Read the model definition and answer for the solid it produces. Units are mm, in the model's axes. Face numbers are marked on the shaded views. A direction names the side the tool comes from. Coordinates: 2 decimals unless noted, no trailing zeros. Loops run counter-clockwise (first coordinate to the right, second up) from the corner with the lowest first, then second, coordinate; pieces in that order, holes last.
Q1. Which of the six approach directions +Z, -Z, +X, -X, +Y, -Y give full straight-line access (tool end or side, diameter ignored) to the marked faces 1 and 2?
Q2. Section B-B (x = 2) is taken. Give the vertices of the cut face in (y, z), then the cut area to 4 significant figures.
Q3. Section A-A (y = 18.25) is taken. Give the vertices of the cut face in (x, z).
Q4. Straight lines are drawn through the part: line 1 (Z direction, x = -17, y = 11.5); line 2 (Z direction, x = -23.5, y = 8); line 3 (X direction, y = 9.25, z = -6.5). For each, find the intervals that lie inside material, in ascending order.
Q5. Section D-D (z = 1.5) is taken. Give the vertices of the cut face in (x, y).
Q6. The mould has two halves that part along X. Classify the marked faces 3, 4, 5 and 6: pulls with the +X half, pulls with the -X half, needs draft (parallel to the pull), parting line crosses it, or undercut.
Q7. Section C-C (x = -15) is taken. Give the vertices of the cut face in (y, z), then the cut area to 4 significant figures.
Q8. Flat-ended cylindrical pins translate along their axes: P1, Ø3, axis at x = 20.5, y = 2, coming from the -Z side; P2, Ø0.9, axis at x = 16, z = -26.5, coming from the +Y side; P3, Ø2.5, axis at y = 12.5, z = -26.5, coming from the +X side. Find the tip coordinate at first contact, or state that the pin passes through.
from build123d import *

# Parameters (mm, degrees)
CROQUIS1_W              = 60
CROQUIS1_H              = 50
SALIENTE_EXTRUIR1_DEPTH = 12.75
CORTAR_EXTRUIR2_START   = 12.75
CROQUIS2_W              = 55
CROQUIS2_H              = 45
CORTAR_EXTRUIR2_DEPTH   = 10.25
SALIENTE_EXTRUIR2_START = 25
CROQUIS4_W              = 49
CROQUIS4_H              = 7.25
SALIENTE_EXTRUIR2_DEPTH = 2.5
SALIENTE_EXTRUIR3_START = -25
CROQUIS4_2_W            = 49
CROQUIS4_2_H            = 7.25
SALIENTE_EXTRUIR3_DEPTH = 2.5
CROQUIS5_W              = 27.5
CROQUIS5_H              = 20
CORTAR_EXTRUIR3_DEPTH   = 10
SALIENTE_EXTRUIR5_START = 25
CROQUIS6_W              = 14
CROQUIS6_H              = 11
SALIENTE_EXTRUIR5_DEPTH = 3
SALIENTE_EXTRUIR6_START = -25
CROQUIS6_2_W            = 14
CROQUIS6_2_H            = 11
SALIENTE_EXTRUIR6_DEPTH = 3
CROQUIS8_W              = 10
CROQUIS8_H              = 1.5
CORTAR_EXTRUIR5_DEPTH   = 43.5
CROQUIS9_W              = 4
CROQUIS9_H              = 8.75
CROQUIS9_W_2            = 6.15
CROQUIS9_H_2            = 6
CORTAR_EXTRUIR6_DEPTH   = 43.5


with BuildPart() as part:
    # Croquis1 → Saliente-Extruir1 (new body)
    with BuildSketch(Plane(origin=(0, 0, 0), x_dir=(1, 0, 0), z_dir=(0, 1, 0))):
        Rectangle(CROQUIS1_W, CROQUIS1_H)
    extrude(amount=SALIENTE_EXTRUIR1_DEPTH)

    # Croquis2 → Cortar-Extruir2 (cut)
    with BuildSketch(Plane(origin=(0, 0, 0), x_dir=(1, 0, 0), z_dir=(0, 1, 0)).offset(CORTAR_EXTRUIR2_START)):
        Rectangle(CROQUIS2_W, CROQUIS2_H)
    extrude(amount=-CORTAR_EXTRUIR2_DEPTH, mode=Mode.SUBTRACT)

    # Croquis4 → Saliente-Extruir2 (add)
    with BuildSketch(Plane.XY.offset(SALIENTE_EXTRUIR2_START)):
        with Locations((0, 16.375)):
            Rectangle(CROQUIS4_W, CROQUIS4_H)
    extrude(amount=-SALIENTE_EXTRUIR2_DEPTH)

    # Croquis4<2> → Saliente-Extruir3 (add)
    with BuildSketch(Plane.XY.offset(SALIENTE_EXTRUIR3_START)):
        with Locations((0, 16.375)):
            Rectangle(CROQUIS4_2_W, CROQUIS4_2_H)
    extrude(amount=SALIENTE_EXTRUIR3_DEPTH)

    # Croquis5 → Cortar-Extruir3 (cut)
    with BuildSketch(Plane(origin=(0, 0, 0), x_dir=(1, 0, 0), z_dir=(0, 1, 0))):
        with Locations((0, -6)):
            Rectangle(CROQUIS5_W, CROQUIS5_H)
    extrude(amount=CORTAR_EXTRUIR3_DEPTH, mode=Mode.SUBTRACT)

    # Croquis6 → Saliente-Extruir5 (add)
    with BuildSketch(Plane.XY.offset(SALIENTE_EXTRUIR5_START)):
        with Locations((-14.25, 10)):
            Rectangle(CROQUIS6_W, CROQUIS6_H)
        with Locations((14.25, 10)):
            Rectangle(CROQUIS6_W, CROQUIS6_H)
    extrude(amount=SALIENTE_EXTRUIR5_DEPTH)

    # Croquis6<2> → Saliente-Extruir6 (add)
    with BuildSketch(Plane.XY.offset(SALIENTE_EXTRUIR6_START)):
        with Locations((-14.25, 10)):
            Rectangle(CROQUIS6_2_W, CROQUIS6_2_H)
        with Locations((14.25, 10)):
            Rectangle(CROQUIS6_2_W, CROQUIS6_2_H)
    extrude(amount=-SALIENTE_EXTRUIR6_DEPTH)

    # Croquis8 → Cortar-Extruir5 (cut)
    with BuildSketch(Plane(origin=(0, 0, 0), x_dir=(1, 0, 0), z_dir=(0, 1, 0))):
        with Locations((-14.25, 25.75)):
            Rectangle(CROQUIS8_W, CROQUIS8_H)
        with Locations((14.25, 25.75)):
            Rectangle(CROQUIS8_W, CROQUIS8_H)
        with Locations((14.25, -25.75)):
            Rectangle(CROQUIS8_W, CROQUIS8_H)
        with Locations((-14.25, -25.75)):
            Rectangle(CROQUIS8_W, CROQUIS8_H)
    extrude(amount=CORTAR_EXTRUIR5_DEPTH, mode=Mode.SUBTRACT)

    # Croquis9 → Cortar-Extruir6 (cut)
    with BuildSketch(Plane(origin=(0, 0, 0), x_dir=(1, 0, 0), z_dir=(0, 1, 0))):
        with Locations((-22.5, -15.125)):
            Rectangle(CROQUIS9_W, CROQUIS9_H)
        with Locations((21.425, -16.5)):
            Rectangle(CROQUIS9_W_2, CROQUIS9_H_2)
    extrude(amount=CORTAR_EXTRUIR6_DEPTH, mode=Mode.SUBTRACT)


solid = part.part
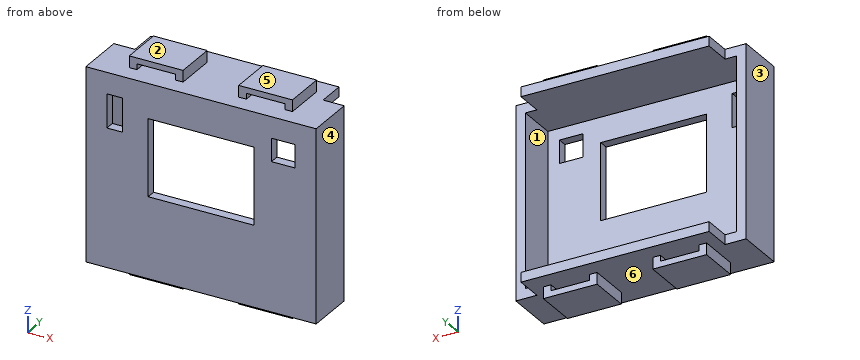
Numbers:
1. face 1: +Y
1. face 2: +Z, +X, -X, +Y, -Y
2. outline: (0, -25) - (20, -25) - (20, -22.5) - (2.5, -22.5) - (2.5, -4) - (0, -4) - close; (0, 16) - (2.5, 16) - (2.5, 22.5) - (20, 22.5) - (20, 25) - (0, 25) - close
2. area: 162.5 mm2
3. outline: (-24.5, -25) - (24.5, -25) - (24.5, -22.5) - (-24.5, -22.5) - close; (-24.5, 22.5) - (24.5, 22.5) - (24.5, 25) - (-24.5, 25) - close
4. line 1: z = -28 to -26.5, -25 to -22.5, 22.5 to 25, 26.5 to 28
4. line 2: z = -25 to -22.5, 22.5 to 25
4. line 3: x = -30 to -27.5, 27.5 to 30
5. outline: (-30, 0) - (-13.75, 0) - (-13.75, 2.5) - (-27.5, 2.5) - (-27.5, 12.75) - (-30, 12.75) - close; (13.75, 0) - (30, 0) - (30, 12.75) - (27.5, 12.75) - (27.5, 2.5) - (13.75, 2.5) - close
6. face 3: pulls with the -X half
6. face 4: pulls with the +X half
6. face 5: needs draft
6. face 6: undercut
7. outline: (0, -25) - (20, -25) - (20, -22.5) - (2.5, -22.5) - (2.5, 22.5) - (20, 22.5) - (20, 25) - (0, 25) - close; (4.5, -28) - (15.5, -28) - (15.5, -26.5) - (4.5, -26.5) - close; (4.5, 26.5) - (15.5, 26.5) - (15.5, 28) - (4.5, 28) - close
7. area: 245.5 mm2
8. P1: stops at z = -25
8. P2: stops at y = 15.5
8. P3: stops at x = 21.25
